from build123d import *

# Parameters (mm, degrees)
SKETCH2_W             = 50
SKETCH2_H             = 130
BOSS_EXTRUDE1_DEPTH   = 9.525
F_4_0MM_DOWEL_HOLE1_D = 4


with BuildPart() as part:
    # Sketch2 → Boss-Extrude1 (new body)
    with BuildSketch(Plane(origin=(0, 0, 0), x_dir=(1, 0, 0), z_dir=(0, 1, 0))):
        Rectangle(SKETCH2_W, SKETCH2_H)
    extrude(amount=BOSS_EXTRUDE1_DEPTH)

    # Ø4.0mm Dowel Hole1 (through all)
    with Locations(Plane(origin=(0, 9.525, 0), x_dir=(1, 0, 0), z_dir=(0, 1, 0))):
        with Locations((16.67, 60.2375), (-16.67, -60.2375), (0, -60.2375), (16.67, -60.2375), (-16.67, 35.7), (0, 35.7), (16.67, 35.7), (-16.67, 60.2375), (0, 60.2375)):
            Hole(F_4_0MM_DOWEL_HOLE1_D / 2)


solid = part.part
The model under review builds one solid part; all positions refer to its coordinate system, in mm. Give positions to 0.01 mm unless a question says otherwise; leave off trailing zeros. Loops run counter-clockwise (first coordinate to the right, second up) from the corner with the lowest first, then second, coordinate; pieces in that order, holes last. Notation, with made-up numbers: (-29.75, 31) -> (-2.75, 31) arc R15 cw to (-2.75, 59) -> close; hole circle Ø9 at (55.25, -0.5). An arc over 180 degrees is marked (long way). Put each result on its own line as item: value. Start each with the question number.
1. Wall thickness on probe 1 along Z at (x, y) = (17, 7); probe 2 along X at (y, z) = (3, -35.7); probe 3 along Z at (x, y) = (-16.67, 7.75): over which ranges is each line inside the solid? List them lowest first.
2. Mouldability with a two-part tool opening along X and no side actions: class faces 1 (the face through (0, 5, 65)), 2 (the face through (25, 5, 1)), 3 (the face through (-0.923, 4.696, -33.926)), 4 (the face through (-25, 5, 1)) as released by +X, released by -X, zero draft, split by the parting line, or undercut.
3. We need section C-C on y = 4.5. State how many separate pieces and enclosed holes the cut face has, then the cut area to 3 significant figures.
4. Clearance check with a flat-ended pin moving along its axis: P1, Ø3, axis at x = -16.67, z = -35.7, coming from the +Y side. State where the tip first meets the part, or that it passes through.
5. We need section B-B on z = -35.7. State the section outline as (x, y) points (3 decimals).
6. We need section A-A on x = -16.67. State the section outline as (y, z) points (1 decimal), then the cut area to 3 significant figures.
Determined:
1. probe 1: -65 to -62.21, -58.26 to -37.67, -33.73 to 58.26, 62.21 to 65
1. probe 2: -25 to -18.67, -14.67 to -2, 2 to 14.67, 18.67 to 25
1. probe 3: -65 to -62.24, -58.24 to -37.7, -33.7 to 58.24, 62.24 to 65
2. face 1: zero draft
2. face 2: released by +X
2. face 3: undercut
2. face 4: released by -X
3. separate pieces: 1
3. enclosed holes: 9
3. area: 6,390 mm^2
4. P1: through
5. outline: (-25, 0) -> (-18.67, 0) -> (-18.67, 9.525) -> (-25, 9.525) -> close; (-14.67, 0) -> (-2, 0) -> (-2, 9.525) -> (-14.67, 9.525) -> close; (2, 0) -> (14.67, 0) -> (14.67, 9.525) -> (2, 9.525) -> close; (18.67, 0) -> (25, 0) -> (25, 9.525) -> (18.67, 9.525) -> close
6. outline: (0, -65) -> (9.5, -65) -> (9.5, -62.2) -> (0, -62.2) -> close; (0, -58.2) -> (9.5, -58.2) -> (9.5, -37.7) -> (0, -37.7) -> close; (0, -33.7) -> (9.5, -33.7) -> (9.5, 58.2) -> (0, 58.2) -> close; (0, 62.2) -> (9.5, 62.2) -> (9.5, 65) -> (0, 65) -> close
6. area: 1,120 mm^2
